Source: CAD feature listing. Evaluate the final solid. Frame: model axes, mm. Face numbers are marked on the shaded views. A direction names the side the tool comes from. Coordinates: 2 decimals unless noted, no trailing zeros. Write each loop counter-clockwise with the first axis right and the second up, starting at its lowest first coordinate (ties: lowest second). Pieces come first, ordered by that corner, then holes. Notation, with made-up numbers: (6, -26.5) -> (27, -26.5) arc R29 cw to (27, 2.5) -> close; hole circle Ø3 at (6, 73). An arc over 180 degrees is marked (long way). One line per item, written item: value. Start each with the question number.
1. Mould query, pull axis X, two halves, no side actions, for the marked faces 5, 6, 7 and 8. Classes: released by +X, released by -X, zero draft, split by the parting line, or undercut.
2. Section query B-B, the plane z = 70.5. Output: boundary loops of the cut face in (x, y), and give its area (3 significant figures).
3. Section query A-A, the plane y = 2. State how many separate pieces and enclosed holes the cut face has, and give its area (3 significant figures).
4. Line query: line 1 (X direction, y = 7.5, z = 65); line 2 (X direction, y = 7, z = 62.5); line 3 (Z direction, x = 63, y = 4). Output: solid intervals per line, ascending.
5. Access query for the marked faces 1, 2, 3 and 4. Directions: +Z, -Z, +X, -X, +Y, -Y. A direction counts if a zero-diameter tool reaches every point of the face in a straight line with its end or side. Return the directions, or none.
6. First-contact query: P1, Ø2, axis at x = 59.5, y = 10, coming from the +Z side; P2, Ø2, axis at y = 1.5, z = 55, coming from the +X side; P3, Ø4, axis at y = 5, z = 55.5, coming from the +X side. Flat tips, straight axial feed; report the tip coordinate or a pass-through.
from build123d import *

# Parameters (mm, degrees)
SKETCH1_R             = 3.2639
BOSS_EXTRUDE1_DEPTH   = 12.7
CHAMFER1_SIZE         = 4.0894
CHAMFER1_SIZE2        = 3.554861186
CHAMFER1_PART_2_SIZE  = 4.0894
CHAMFER1_PART_2_SIZE2 = 3.554861186
CUT_EXTRUDE1_DEPTH    = 13.7000001


with BuildPart() as part:
    # Sketch1 → Boss-Extrude1 (new body)
    with BuildSketch(Plane(origin=(0, 0, 0), x_dir=(1, 0, 0), z_dir=(0, 1, 0))):
        with BuildLine():
            Line((98.733031573, -68.985835228), (100.942599672, -71.978006872))
            ThreePointArc((100.942599672, -71.978006872), (102.740427245, -73.495514847), (105.029143887, -74.040299732))
            Line((105.029143887, -74.040299732), (124.201892168, -74.040299732))
            ThreePointArc((124.201892168, -74.040299732), (129.062693158, -70.745465469), (127.802444272, -65.010041176))
            Line((127.802444272, -65.010041176), (106.094318665, -44.426787292))
            Line((106.094318665, -44.426787292), (103.19820861, -45.713487798))
            Line((103.19820861, -45.713487798), (68.977352979, -45.713487798))
            Line((68.977352979, -45.713487798), (61.792374607, -42.131557151))
            Line((61.792374607, -42.131557151), (24.038270246, -62.563232545))
            ThreePointArc((24.038270246, -62.563232545), (21.322907648, -65.331673968), (20.915380805, -69.188017292))
            add(Edge.make_bspline(
                [(62.315611289, -66.923542367), (58.569118303, -55.043460273), (51.499770267, -53.452589153), (20.915380805, -69.188017292)],
                knots=[0, 0, 0, 0, 1, 1, 1, 1], degree=3))
            Line((62.315611289, -66.923542367), (94.646487358, -66.923542367))
            ThreePointArc((94.646487358, -66.923542367), (96.935204, -67.468327252), (98.733031573, -68.985835228))
        make_face()
        with Locations((60.150170667, -51.891201826)):
            Circle(SKETCH1_R, mode=Mode.SUBTRACT)
        with Locations((71.3764156, -59.641849895)):
            Circle(SKETCH1_R, mode=Mode.SUBTRACT)
        with Locations((84.237729699, -53.077081169)):
            Circle(SKETCH1_R, mode=Mode.SUBTRACT)
        with Locations((96.63028976, -60.633621731)):
            Circle(SKETCH1_R, mode=Mode.SUBTRACT)
    extrude(amount=BOSS_EXTRUDE1_DEPTH)

    # Chamfer1
    chamfer1_edges = [part.edges().sort_by_distance(p)[0] for p in [
        (56.886270667, 12.7, 51.891201826),
    ]]
    chamfer1_side = [part.faces().sort_by_distance(p)[0] for p in [
        (56.886270667, 6.35, 51.891201826),
    ]]
    chamfer(chamfer1_edges, length=CHAMFER1_SIZE, length2=CHAMFER1_SIZE2, reference=chamfer1_side[0])

    # Chamfer1 part 2
    chamfer1_part_2_edges = [part.edges().sort_by_distance(p)[0] for p in [
        (80.973829699, 12.7, 53.077081169),
    ]]
    chamfer1_part_2_side = [part.faces().sort_by_distance(p)[0] for p in [
        (80.973829699, 6.35, 53.077081169),
    ]]
    chamfer(chamfer1_part_2_edges, length=CHAMFER1_PART_2_SIZE, length2=CHAMFER1_PART_2_SIZE2, reference=chamfer1_part_2_side[0])

    # Sketch2 → Cut-Extrude1 (cut, through all)
    with BuildSketch(Plane(origin=(0, 12.7, 0), x_dir=(1, 0, 0), z_dir=(0, 1, 0))):
        Polygon((77.89856543, -59.263365519), (74.30971343, -53.804260267), (67.7875636, -54.182744643), (64.85426577, -60.020334272), (68.443117769, -65.479439524), (74.9652676, -65.100955148), align=None)
        Polygon((103.042754495, -61.883415654), (100.918875415, -55.705161331), (94.50641068, -54.455367408), (90.217825025, -59.383827808), (92.341704106, -65.562082131), (98.754168841, -66.811876054), align=None)
    extrude(amount=-CUT_EXTRUDE1_DEPTH, mode=Mode.SUBTRACT)


solid = part.part
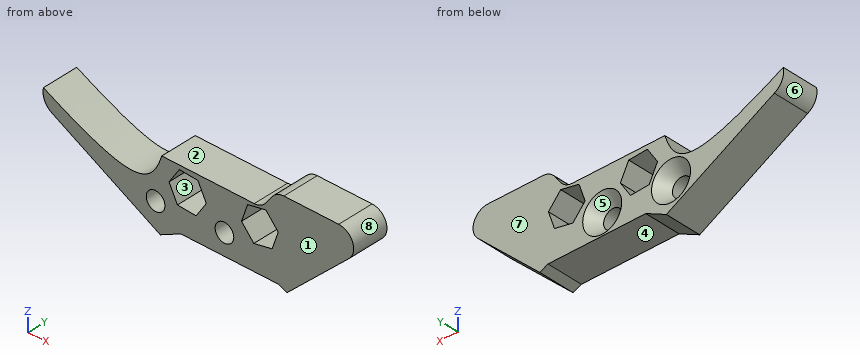
Computed values:
1. face 5: undercut
1. face 6: released by -X
1. face 7: zero draft
1. face 8: released by +X
2. outline: (99.85, 0) -> (129.15, 0) -> (129.15, 12.7) -> (99.85, 12.7) -> close
2. area: 372 mm²
3. separate pieces: 1
3. enclosed holes: 4
3. area: 1,480 mm²
4. line 1: x = 21.49 to 29.36, 61.64 to 68.13, 75.02 to 92.15, 100.33 to 127.79
4. line 2: x = 24.16 to 34.88, 60.46 to 66.48, 76.27 to 91.29, 102.51 to 125.16
4. line 3: z = 42.73 to 50.3, 53.48 to 66.92
5. face 1: +Z, -Z, +X, -X, -Y
5. face 2: +Z, +Y, -Y
5. face 3: +Y, -Y
5. face 4: -Z, +Y, -Y
6. P1: stops at z = 62.57
6. P2: stops at x = 118.3
6. P3: stops at x = 119.88
